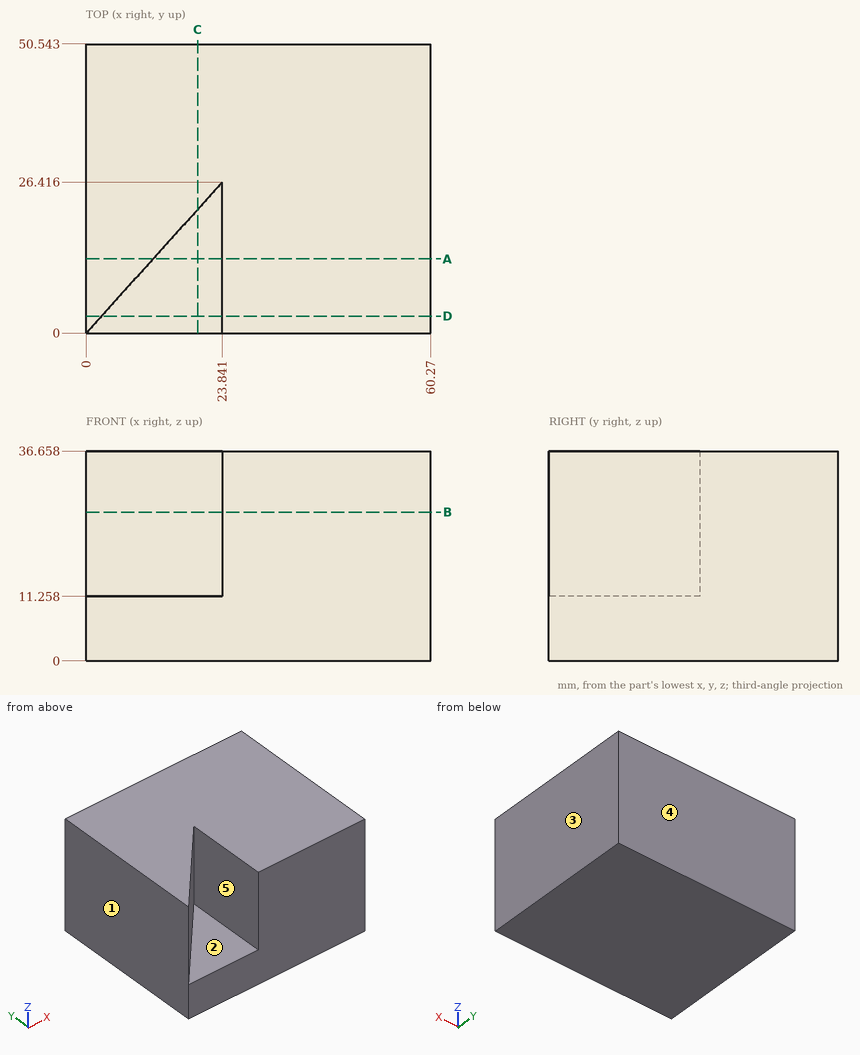
Geometry check sheet. Reference: drawing and pictorial views, mm from the part's lowest x, y, z. A direction names the side the tool comes from. Round coordinates to 2 decimals unless told otherwise and drop trailing zeros. Order: outer loops, then holes, each group sorted by start corner. A loop starts at its lowest first (then second) coordinate and runs counter-clockwise, first axis right, second up. Notation, with made-up numbers: (-14, -13) - (39, -13) arc R11 ccw to (39, -7) - close; hole circle Ø3 at (52.25, 2.5). An arc over 180 degrees is marked (long way). One line per question, with ' | ' between items. Start each with the question number.
(1) Sectioned sample at B-B on z = 26. Record the cut outline in (x, y), and give its area (3 significant figures).
(2) Release check for a two-part mould opening along X. For the marked faces 1, 2 and 3 record: released by +X, released by -X, zero draft, split by the parting line, or undercut.
(3) Sectioned sample at D-D on y = 3. Record the cut outline in (x, z), and give its area (3 significant figures).
(4) Sectioned sample at A-A on y = 13. Record the cut outline in (x, z), and give its area (3 significant figures).
(5) Thickness scan on L1, parallel to Z at x = 15.5, y = 3; L2, parallel to X at y = 19.5, z = 30; L3, parallel to X at y = 13, z = 13.5. Record the ranges inside material, lowest first. Write a range as [from, to].
(6) Sectioned sample at C-C on x = 19.5. Record the cut outline in (y, z).
(7) Access from +Z, -Z, +X, -X, +Y, -Y to the whole of each face (thin tool, end or side, straight path). Record for the marked faces 4 and 5.
(8) Depth check by flat-ended pin: pin 1 Ø5 at (x, y) = (12, 43.5) entering from -Z; pin 2 Ø12 at (x, y) = (16.5, 8) entering from +Z. Enter the tip coordinate at first touch or a pass-through.
Conclusion:
1) outline: (0, 0) - (23.84, 26.42) - (23.84, 0) - (60.27, 0) - (60.27, 50.54) - (0, 50.54) - close | area: 2,730 mm2
2) face 1: released by -X | face 2: undercut | face 3: released by +X
3) outline: (0, 0) - (60.27, 0) - (60.27, 36.66) - (23.84, 36.66) - (23.84, 11.26) - (2.71, 11.26) - (2.71, 36.66) - (0, 36.66) - close | area: 1,670 mm2
4) outline: (0, 0) - (60.27, 0) - (60.27, 36.66) - (23.84, 36.66) - (23.84, 11.26) - (11.73, 11.26) - (11.73, 36.66) - (0, 36.66) - close | area: 1,900 mm2
5) L1: z = [0, 11.26] | L2: x = [0, 17.6], [23.84, 60.27] | L3: x = [0, 11.73], [23.84, 60.27]
6) outline: (0, 0) - (50.54, 0) - (50.54, 36.66) - (21.61, 36.66) - (21.61, 11.26) - (0, 11.26) - close
7) face 4: +Z, -Z, +X, -X, +Y | face 5: +Z, -Y
8) pin 1: stops at z = 0 | pin 2: stops at z = 11.26
